```python
from build123d import *
from OCP.BRepFilletAPI import BRepFilletAPI_MakeChamfer

# Parameters (mm, degrees)
CROQUIS1_W              = 150
CROQUIS1_H              = 120
SALIENTE_EXTRUIR1_DEPTH = 10
CROQUIS2_W              = 143
CROQUIS2_H              = 113
SALIENTE_EXTRUIR2_DEPTH = 3
CORTAR_EXTRUIR4_DEPTH   = 10
CROQUIS5_W              = 20
CROQUIS5_H              = 20
CORTAR_EXTRUIR5_DEPTH   = 3
CROQUIS7_R              = 2
CORTAR_EXTRUIR6_DEPTH   = 97.566039579
CHAFL_N1_SIZE           = 4
CHAFL_N1_SIZE2          = 2.309401077
REDONDEO3_R             = 4
REDONDEO4_R             = 4
REDONDEO5_R             = 1
CROQUIS8_R              = 2.5
CROQUIS8_R_2            = 5.5
CROQUIS8_W              = 21.5
CROQUIS8_H              = 31
CROQUIS8_W_2            = 30
CROQUIS8_H_2            = 11
CORTAR_EXTRUIR7_DEPTH   = 97.922649572
CORTAR_EXTRUIR8_DEPTH   = 0.5


with BuildPart() as part:
    # Croquis1 → Saliente-Extruir1 (new body)
    with BuildSketch(Plane(origin=(0, 0, 0), x_dir=(1, 0, 0), z_dir=(0, 1, 0))):
        Rectangle(CROQUIS1_W, CROQUIS1_H)
    extrude(amount=SALIENTE_EXTRUIR1_DEPTH)

    # Croquis2 → Saliente-Extruir2 (add)
    with BuildSketch(Plane(origin=(0, 10, 0), x_dir=(1, 0, 0), z_dir=(0, 1, 0))):
        Rectangle(CROQUIS2_W, CROQUIS2_H)
    extrude(amount=SALIENTE_EXTRUIR2_DEPTH)

    # Croquis4 → Cortar-Extruir4 (cut)
    with BuildSketch(Plane(origin=(0, 13, 0), x_dir=(1, 0, 0), z_dir=(0, 1, 0))):
        Polygon((-65, 54), (65, 54), (65, 50), (69, 50), (69, -50), (65, -50), (65, -54), (-65, -54), (-65, -50), (-69, -50), (-69, 50), (-65, 50), align=None)
    extrude(amount=-CORTAR_EXTRUIR4_DEPTH, mode=Mode.SUBTRACT)

    # Croquis5 → Cortar-Extruir5 (cut)
    with BuildSketch(Plane(origin=(0, 13, 0), x_dir=(1, 0, 0), z_dir=(0, 1, 0))):
        with Locations((-65, 50)):
            Rectangle(CROQUIS5_W, CROQUIS5_H)
        with Locations((65, 50)):
            Rectangle(CROQUIS5_W, CROQUIS5_H)
        with Locations((65, -50)):
            Rectangle(CROQUIS5_W, CROQUIS5_H)
        with Locations((-65, -50)):
            Rectangle(CROQUIS5_W, CROQUIS5_H)
    extrude(amount=-CORTAR_EXTRUIR5_DEPTH, mode=Mode.SUBTRACT)

    # Croquis7 → Cortar-Extruir6 (cut, through all)
    with BuildSketch(Plane(origin=(0, 10, 0), x_dir=(1, 0, 0), z_dir=(0, 1, 0))):
        with Locations(Location((-70, 55, 0), (0, 0, 270))):
            Circle(CROQUIS7_R)
        with Locations(Location((70, 55, 0), (0, 0, 270))):
            Circle(CROQUIS7_R)
        with Locations(Location((70, -55, 0), (0, 0, 270))):
            Circle(CROQUIS7_R)
        with Locations(Location((-70, -55, 0), (0, 0, 270))):
            Circle(CROQUIS7_R)
    extrude(amount=-CORTAR_EXTRUIR6_DEPTH, mode=Mode.SUBTRACT)

    # Chaflán1: one chamfer whose edges measure the first distance from different faces: ONE call of the kernel's chamfer builder (chamfer() names one face for all edges)
    chafl_n1_edges_1 = [part.edges().sort_by_distance(p)[0] for p in [
        (70, 0, 53),
    ]]
    chafl_n1_side_1 = [part.faces().sort_by_distance(p)[0] for p in [
        (70, 5, 53),
    ]]
    chafl_n1_edges_2 = [part.edges().sort_by_distance(p)[0] for p in [
        (-70, 0, -57),
    ]]
    chafl_n1_side_2 = [part.faces().sort_by_distance(p)[0] for p in [
        (-70, 5, -57),
    ]]
    chafl_n1_edges_3 = [part.edges().sort_by_distance(p)[0] for p in [
        (-70, 0, 53),
    ]]
    chafl_n1_side_3 = [part.faces().sort_by_distance(p)[0] for p in [
        (-70, 5, 53),
    ]]
    chafl_n1_edges_4 = [part.edges().sort_by_distance(p)[0] for p in [
        (70, 0, -57),
    ]]
    chafl_n1_side_4 = [part.faces().sort_by_distance(p)[0] for p in [
        (70, 5, -57),
    ]]
    chafl_n1 = BRepFilletAPI_MakeChamfer(part.part.solid().wrapped)
    for e in chafl_n1_edges_1:
        chafl_n1.Add(CHAFL_N1_SIZE, CHAFL_N1_SIZE2, e.wrapped, chafl_n1_side_1[0].wrapped)  # the first distance lies on this face
    for e in chafl_n1_edges_2:
        chafl_n1.Add(CHAFL_N1_SIZE, CHAFL_N1_SIZE2, e.wrapped, chafl_n1_side_2[0].wrapped)  # the first distance lies on this face
    for e in chafl_n1_edges_3:
        chafl_n1.Add(CHAFL_N1_SIZE, CHAFL_N1_SIZE2, e.wrapped, chafl_n1_side_3[0].wrapped)  # the first distance lies on this face
    for e in chafl_n1_edges_4:
        chafl_n1.Add(CHAFL_N1_SIZE, CHAFL_N1_SIZE2, e.wrapped, chafl_n1_side_4[0].wrapped)  # the first distance lies on this face
    add(Compound.cast(chafl_n1.Shape()), mode=Mode.REPLACE)

    # Redondeo3
    redondeo3_edges = [part.edges().sort_by_distance(p)[0] for p in [
        (75, 5, 60),
        (-75, 5, 60),
        (-75, 5, -60),
        (75, 5, -60),
    ]]
    fillet(redondeo3_edges, radius=REDONDEO3_R)

    # Redondeo4
    redondeo4_edges = [part.edges().sort_by_distance(p)[0] for p in [
        (65, 6.5, -50),
        (65, 6.5, 50),
        (-65, 6.5, 50),
        (-65, 6.5, -50),
    ]]
    fillet(redondeo4_edges, radius=REDONDEO4_R - 0.0001)  # a hair under: the kernel refuses the full size

    # Redondeo5
    redondeo5_edges = [part.edges().sort_by_distance(p)[0] for p in [
        (70.25, 13, 40),
        (55, 13, 55.25),
        (55, 13, -55.25),
        (70.25, 13, -40),
        (-55, 13, -55.25),
        (-70.25, 13, -40),
        (0, 13, -54),
        (69, 13, 0),
        (0, 13, 54),
        (-69, 13, 0),
        (71.5, 13, 0),
        (0, 13, -56.5),
        (-71.5, 13, 0),
        (0, 13, 56.5),
        (-55, 13, 55.25),
        (-70.25, 13, 40),
    ]]
    fillet(redondeo5_edges, radius=REDONDEO5_R)

    # Croquis8 → Cortar-Extruir7 (cut, through all)
    with BuildSketch(Plane.XZ):
        with Locations(Location((0, 0, 0), (0, 0, 270))):
            Circle(CROQUIS8_R)
        with Locations(Location((55, 0, 0), (0, 0, 270))):
            Circle(CROQUIS8_R_2)
        with Locations((-34.25, 0)):
            Rectangle(CROQUIS8_W, CROQUIS8_H)
        with Locations((0, 40)):
            Rectangle(CROQUIS8_W_2, CROQUIS8_H_2)
    extrude(amount=-CORTAR_EXTRUIR7_DEPTH, mode=Mode.SUBTRACT)

    # Croquis9 → Cortar-Extruir8 (cut)
    with BuildSketch(Plane.XZ):
        Polygon((-23.5, 2.5), (-23.5, -2.5), (-12.5, -2.5), (-12.5, -12.5), (12.5, -12.5), (12.5, -2.5), (50.101020514, -2.5), (50.101020514, 2.5), (20.5, 2.5), (20.5, 42.5), (-20.5, 42.5), (-20.5, 2.5), align=None)
        Polygon((-12.5, 2.5), (-12.5, 12.5), (12.5, 12.5), (12.5, 2.5), (15.5, 2.5), (15.5, 37.5), (-15.5, 37.5), (-15.5, 2.5), align=None, mode=Mode.SUBTRACT)
    extrude(amount=-CORTAR_EXTRUIR8_DEPTH, mode=Mode.SUBTRACT)


solid = part.part
```
Verification items for the finished model (mm, model axes). A direction names the side the tool comes from. Give positions to 0.01 mm unless a question says otherwise; leave off trailing zeros. Order: outer loops, then holes, each group sorted by start corner. A loop starts at its lowest first (then second) coordinate and runs counter-clockwise, first axis right, second up. Notation, with made-up numbers: M 40.5,0.25 L 56.5,0.25 A17 cw 56.5,23.25 Z; hole C 20,-26 d10. An arc over 180 degrees is marked long. Return JSON: item names as keys, results as strings. Group by question number.
1) Go/stop test with flat-tipped pins: pin 1 Ø3 at (x, z) = (54.5, -39.5) entering from +Y; pin 2 Ø4.5 at (x, z) = (70, -55) entering from +Y; pin 3 Ø2 at (x, y) = (-70, 11.5) entering from +Z. Record where each tip stops, or that it passes through.
2) Section check D-D on y = 6.75. Give the number of separate pieces and of enclosed holes in the cut face, and give its area (3 significant figures).
3) Section check C-C on x = -27. Record the cut outline in (y, z).
4) Section check B-B on x = 0. Record the cut outline in (y, z), and give its area (3 significant figures).
5) Section check A-A on z = 0. Record the cut outline in (x, y), and give its area (3 significant figures).
6) Mould release check, pull along X, two halves, no side actions. Record for faces 1 (the face through (-34, 1, 15.5)), 2 (the face through (-1, 5, 60)), 3 (the face through (-73.859, 5.07, -58.797)), 4 (the face through (-23.5, 1, 0)): pulls with the +X half, pulls with the -X half, needs draft (parallel to the pull), parting line crosses it, or undercut.
7) Scan lines: line 1 (X direction, y = 7.35, z = -55); line 2 (X direction, y = 2.25, z = 0); line 3 (Z direction, x = 55, y = 1.2). Record each from-to range of solid material in increasing order.
8) Access from +Z, -Z, +X, -X, +Y, -Y to the whole of each face (thin tool, end or side, straight path). Record for faces 5 (the face through (75, 5, 1)), 6 (the face through (-69, 8, 1)), 7 (the face through (0, 1, 45.5)).
Answer block:
{
 "1": {"pin 1": "stops at y = 3", "pin 2": "stops at y = 10", "pin 3": "stops at z = 40"},
 "2": {"separate pieces": "1", "enclosed holes": "5", "area": "3,080 mm^2"},
 "3": {"outline": "M 0,-60 L 10,-60 L 10,-56.5 L 12,-56.5 A1 ccw 13,-55.5 L 13,-55 A1 ccw 12,-54 L 3,-54 L 3,-15.5 L 0,-15.5 Z; M 0,15.5 L 3,15.5 L 3,54 L 12,54 A1 ccw 13,55 L 13,55.5 A1 ccw 12,56.5 L 10,56.5 L 10,60 L 0,60 Z"},
 "4": {"outline": "M 0,-60 L 10,-60 L 10,-56.5 L 12,-56.5 A1 ccw 13,-55.5 L 13,-55 A1 ccw 12,-54 L 3,-54 L 3,-2.5 L 0.5,-2.5 L 0.5,-12.5 L 0,-12.5 Z; M 0,12.5 L 0.5,12.5 L 0.5,2.5 L 3,2.5 L 3,34.5 L 0,34.5 Z; M 0,45.5 L 3,45.5 L 3,54 L 12,54 A1 ccw 13,55 L 13,55.5 A1 ccw 12,56.5 L 10,56.5 L 10,60 L 0,60 Z", "area": "400 mm^2"},
 "5": {"outline": "M -75,0 L -45,0 L -45,3 L -69,3 L -69,12 A1 ccw -70,13 L -70.5,13 A1 ccw -71.5,12 L -71.5,10 L -75,10 Z; M -23.5,0.5 L -2.5,0.5 L -2.5,3 L -23.5,3 Z; M 2.5,0.5 L 49.5,0.5 L 49.5,3 L 2.5,3 Z; M 60.5,0 L 75,0 L 75,10 L 71.5,10 L 71.5,12 A1 ccw 70.5,13 L 70,13 A1 ccw 69,12 L 69,3 L 60.5,3 Z", "area": "402 mm^2"},
 "6": {"face 1": "undercut", "face 2": "needs draft", "face 3": "pulls with the -X half", "face 4": "undercut"},
 "7": {"line 1": "x = -75 to -72, -68 to 68, 72 to 75", "line 2": "x = -75 to -45, -23.5 to -2.5, 2.5 to 49.5, 60.5 to 75", "line 3": "z = -60 to -5.5, 5.5 to 60"},
 "8": {"face 5": "+Z, -Z, +X, +Y, -Y", "face 6": "+Y", "face 7": "+Y, -Y"}
}
